```python
from build123d import *

# Parameters (mm, degrees)
SKETCH1_W               = 8
SKETCH1_H               = 8
BOSS_EXTRUDE1_DEPTH     = 3
CUT_EXTRUDE1_DEPTH      = 12.704699911
CUT_EXTRUDE1_DEPTH_BACK = 12.704699911
CUT_EXTRUDE2_DEPTH      = 11
SKETCH4_R               = 1.8
CUT_EXTRUDE3_DEPTH      = 0.8
SKETCH5_W               = 8
SKETCH5_H               = 1
BOSS_EXTRUDE2_DEPTH     = 2
FILLET1_R               = 4
CUT_EXTRUDE4_DEPTH      = 0.4


with BuildPart() as part:
    # Sketch1 → Boss-Extrude1 (new body)
    with BuildSketch(Plane(origin=(0, 0, 0), x_dir=(1, 0, 0), z_dir=(0, 1, 0))):
        with Locations((4, 4)):
            Rectangle(SKETCH1_W, SKETCH1_H)
    extrude(amount=BOSS_EXTRUDE1_DEPTH)

    # Sketch2 → Cut-Extrude1 (cut, two sides: drawn at the far end of the back side and taken through both)
    with BuildSketch(Plane.XY.offset(-CUT_EXTRUDE1_DEPTH_BACK)):
        Polygon((0, 0), (0.6, 3), (0, 3), align=None)
        Polygon((8, 0), (7.4, 3), (8, 3), align=None)
    extrude(amount=CUT_EXTRUDE1_DEPTH + CUT_EXTRUDE1_DEPTH_BACK, mode=Mode.SUBTRACT)

    # Sketch3 → Cut-Extrude2 (cut)
    with BuildSketch(Plane(origin=(0, 0, 0), x_dir=(0, 0, -1), z_dir=(1, 0, 0))):
        Polygon((0, 0), (0.6, 3), (0, 3), align=None)
        Polygon((8, 3), (7.4, 3), (8, 0), align=None)
    extrude(amount=CUT_EXTRUDE2_DEPTH, mode=Mode.SUBTRACT)

    # Sketch4 → Cut-Extrude3 (cut)
    with BuildSketch(Plane.XZ):
        with Locations(Location((4, -3.75, 0), (0, 0, 270))):
            Circle(SKETCH4_R)
    extrude(amount=-CUT_EXTRUDE3_DEPTH, mode=Mode.SUBTRACT)

    # Sketch5 → Boss-Extrude2 (add)
    with BuildSketch(Plane.XZ):
        with Locations((4, -7.5)):
            Rectangle(SKETCH5_W, SKETCH5_H)
    extrude(amount=BOSS_EXTRUDE2_DEPTH)

    # Fillet1
    # the kernel refuses this fillet: 4 mm, written as the material it takes off along each edge
    with BuildSketch(Plane(origin=(8, -2, -16.660254038), x_dir=(0, 1, 0), z_dir=(0, 0, 1)), Plane(origin=(0, -2, 1.660254038), x_dir=(0, 1, 0), z_dir=(0, 0, -1))) as fillet1_piece_1:
        with BuildLine():
            CenterArc((4, 3.464101615), FILLET1_R, 180, 60)
            Line((0, 3.464101615), (-0.08, 3.464101615))
            Line((-0.08, 3.464101615), (-0.08, 0))
            Line((-0.08, 0), (0, -0.08))
            ThreePointArc((0, -0.08), (1, -0.08), (1.96, -0.069282032))
            Line((1.96, -0.069282032), (2, 0))
        make_face()
    extrude(amount=18.320508076, mode=Mode.SUBTRACT)

    # Sketch6 → Cut-Extrude4 (cut)
    with BuildSketch(Plane(origin=(0, 3, 0), x_dir=(1, 0, 0), z_dir=(0, 1, 0))):
        Polygon((2.33946821, 2.056832464), (2.33946821, 2.774781182), (4.546198979, 5.390165797), (2.595878466, 5.390165797), (2.595878466, 6.056832464), (5.518955389, 6.056832464), (5.518955389, 5.390165797), (3.268154107, 2.72349913), (5.570237441, 2.72349913), (5.570237441, 2.056832464), align=None)
    extrude(amount=-CUT_EXTRUDE4_DEPTH, mode=Mode.SUBTRACT)


solid = part.part
```
Check sheet for the modelled part. Datum: model origin and axes. Units: mm. A direction names the side the tool comes from. Round coordinates to 2 decimals unless told otherwise and drop trailing zeros. Order: outer loops, then holes, each group sorted by start corner. A loop starts at its lowest first (then second) coordinate and runs counter-clockwise, first axis right, second up. Notation, with made-up numbers: (70, -40) -> (120, -40) arc R16 cw to (120, -12) -> close; hole circle Ø3 at (60, 59). An arc over 180 degrees is marked (long way). Use CSV: the item, a comma, the result in double quotes.
(1) Draft check along Z on faces 5 (the face through (4, 2.6, -4)), 6 (the face through (4, -1, -8)), 7 (the face through (3.9, 1.5, -0.3)), 8 (the face through (0.3, 1.5, -4.1)). Enter one of: pulls with the +Z half, pulls with the -Z half, needs draft (parallel to the pull), parting line crosses it, or undercut.
Worked out:
face 5,"undercut"
face 6,"pulls with the -Z half"
face 7,"pulls with the +Z half"
face 8,"needs draft"
(2) Tool access check on faces 1 (the face through (3, 0, -2)), 2 (the face through (4, 0.8, -4)), 3 (the face through (6.51, -1.48, -7.51)), 4 (the face through (3.427, 2.803, -4.064)). Record the directions out of +Z, -Z, +X, -X, +Y, -Y that give a thin tool (end or side, any length) a straight path to the whole face; none if there is none.
Worked out:
face 1,"+Z, +X, -X, -Y"
face 2,"-Y"
face 3,"+Z, -Z, +X, -Y"
face 4,"+Y"
(3) Cross-section at B-B (x = 6.5). Record the boundary of the cut face in (y, z), and give its area (3 significant figures).
Worked out:
outline,"(-1.48, -8) -> (0, -8) -> (3, -7.4) -> (3, -0.6) -> (0, 0) -> (0, -7) -> (-1.48, -7) -> close"
area,"23.7 mm²"
(4) Cross-section at C-C (z = -3.25). Record the boundary of the cut face in (x, y), and give its area (3 significant figures).
Worked out:
outline,"(0, 0) -> (2.27, 0) -> (2.27, 0.8) -> (5.73, 0.8) -> (5.73, 0) -> (8, 0) -> (7.4, 3) -> (3.71, 3) -> (3.71, 2.6) -> (2.74, 2.6) -> (2.74, 3) -> (0.6, 3) -> close"
area,"19.0 mm²"
(5) Cross-section at A-A (z = -5.75). Record the boundary of the cut face in (x, y), and give its area (3 significant figures).
Worked out:
outline,"(0, 0) -> (8, 0) -> (7.4, 3) -> (5.52, 3) -> (5.52, 2.6) -> (2.6, 2.6) -> (2.6, 3) -> (0.6, 3) -> close"
area,"21.0 mm²"
(6) Material ranges on line 1 along Y through (x, z) = (6.25, -4.25); line 2 along X through (y, z) = (0.5, -3.75); line 3 along Z through (x, y) = (5.25, 0.4), recorded low to high. Write a range as from..to.
Worked out:
line 1,"0..3"
line 2,"0.1..2.2, 5.8..7.9"
line 3,"-7.92..-5.05, -2.45..-0.08"
(7) Depth check by flat-ended pin: pin 1 (1.1 mm diameter, centred on x = 4.5, z = -3.5, fed in from -Y); pin 2 (0.6 mm diameter, centred on x = 4.5, y = -1.5, fed in from +Z); pin 3 (3.5 mm diameter, centred on x = 2.5, z = -3.5, fed in from -Y); pin 4 (1 mm diameter, centred on y = -1, z = -4.5, fed in from -X). Enter the tip coordinate at first touch or a pass-through.
Worked out:
pin 1,"y = 0.8"
pin 2,"z = -7"
pin 3,"y = 0"
pin 4,"through"
(8) Cross-section at D-D (x = 4). Record the boundary of the cut face in (y, z), and give its area (3 significant figures).
Worked out:
outline,"(-2, -8) -> (0, -8) -> (3, -7.4) -> (3, -6.06) -> (2.6, -6.06) -> (2.6, -5.39) -> (3, -5.39) -> (3, -4.74) -> (2.6, -4.74) -> (2.6, -3.59) -> (3, -3.59) -> (3, -2.72) -> (2.6, -2.72) -> (2.6, -2.06) -> (3, -2.06) -> (3, -0.6) -> (0, 0) -> (0, -1.95) -> (0.8, -1.95) -> (0.8, -5.55) -> (0, -5.55) -> (0, -7) -> (-2, -7) -> close"
area,"20.3 mm²"
